from build123d import *

# Parameters (mm, degrees)
CROQUIS1_W              = 150
CROQUIS1_H              = 90
SALIENTE_EXTRUIR1_DEPTH = 5
SALIENTE_EXTRUIR2_DEPTH = 3
CROQUIS2_R              = 2.5
CORTAR_EXTRUIR1_DEPTH   = 10


with BuildPart() as part:
    # Croquis1 → Saliente-Extruir1 (new body)
    with BuildSketch(Plane(origin=(0, 0, 0), x_dir=(1, 0, 0), z_dir=(0, 1, 0))):
        Rectangle(CROQUIS1_W, CROQUIS1_H)
    extrude(amount=SALIENTE_EXTRUIR1_DEPTH)

    # Croquis1<3> → Saliente-Extruir2 (add)
    with BuildSketch(Plane(origin=(0, 0, 0), x_dir=(1, 0, 0), z_dir=(0, 1, 0))):
        Polygon((-75, -45), (-75, 45), (75, 45), (75, -45), (95, -45), (95, 65), (-95, 65), (-95, -45), align=None)
    extrude(amount=SALIENTE_EXTRUIR2_DEPTH)

    # Croquis2 → Cortar-Extruir1 (cut)
    with BuildSketch(Plane.XZ):
        with Locations((85, 30)):
            Circle(CROQUIS2_R)
        with Locations((70, -55)):
            Circle(CROQUIS2_R)
        with Locations((-85, -40)):
            Circle(CROQUIS2_R)
        with Locations((-85, -5)):
            Circle(CROQUIS2_R)
        with Locations((-85, 30)):
            Circle(CROQUIS2_R)
        with Locations((0, -55)):
            Circle(CROQUIS2_R)
        with Locations((-70, -55)):
            Circle(CROQUIS2_R)
        with Locations((85, -5)):
            Circle(CROQUIS2_R)
        with Locations((85, -40)):
            Circle(CROQUIS2_R)
    extrude(amount=-CORTAR_EXTRUIR1_DEPTH, mode=Mode.SUBTRACT)


solid = part.part
Read the model definition and answer for the solid it produces. Units are mm, in the model's axes. Give positions to 0.01 mm unless a question says otherwise; leave off trailing zeros. Write each loop counter-clockwise with the first axis right and the second up, starting at its lowest first coordinate (ties: lowest second). Pieces come first, ordered by that corner, then holes. Notation, with made-up numbers: (57.5, 89) -> (101.5, 89) arc R4 ccw to (101.5, 94) -> close; hole circle Ø3 at (-37, 3). An arc over 180 degrees is marked (long way). Answer as a JSON object with one key per item and string values. Group by question number.
1) Consider L1, parallel to Z at x = -85, y = 1.2; L2, parallel to Z at x = -70, y = 2; L3, parallel to Y at x = -51.5, z = -57.5. Determine where each line is inside the solid, lowest interval first. Write a range as from..to.
2) Each of these flat-tipped pins is pushed along its axis until it touches: P1, Ø1.6, axis at y = 4.5, z = -18, coming from the +X side; P2, Ø4.5, axis at x = 85, z = -5, coming from the -Y side; P3, Ø0.6, axis at y = 3.5, z = 4, coming from the -X side; P4, Ø6, axis at x = -85, z = -5, coming from the +Y side. Where does it stop, or does it pass through?
3) Find section D-D (x = -29). Write down the section's boundary in (y, z).
4) Find section B-B (x = 85). Write down the section's boundary in (y, z), and give its area (3 significant figures).
5) The mould has two halves that part along Z. Classify faces 1 (the cylindrical face through (83, 1.5, -41.5)), 2 (the flat face through (-1, 3, -47)), 3 (the cylindrical face through (-87.5, 1.5, -4.9)), 4 (the flat face through (-1, 2, 45)): +Z half, -Z half, draft (parallel to the pull), parting line (faces both ways), or undercut.
6) Find section A-A (z = -55). Write down the section's boundary in (x, y), and give its area (3 significant figures).
7) Find section C-C (z = 30). Write down the section's boundary in (x, y), and give its area (3 significant figures).
Values follow:
{
 "1": {"L1": "z = -65..-42.5, -37.5..-7.5, -2.5..27.5, 32.5..45", "L2": "z = -65..-57.5, -52.5..45", "L3": "y = 0..3"},
 "2": {"P1": "stops at x = 75", "P2": "passes through", "P3": "stops at x = -75", "P4": "stops at y = 3"},
 "3": {"outline": "(0, -65) -> (3, -65) -> (3, -45) -> (5, -45) -> (5, 45) -> (0, 45) -> close"},
 "4": {"outline": "(0, -65) -> (3, -65) -> (3, -42.5) -> (0, -42.5) -> close; (0, -37.5) -> (3, -37.5) -> (3, -7.5) -> (0, -7.5) -> close; (0, -2.5) -> (3, -2.5) -> (3, 27.5) -> (0, 27.5) -> close; (0, 32.5) -> (3, 32.5) -> (3, 45) -> (0, 45) -> close", "area": "285 mm2"},
 "5": {"face 1": "undercut", "face 2": "draft", "face 3": "undercut", "face 4": "+Z half"},
 "6": {"outline": "(-95, 0) -> (-72.5, 0) -> (-72.5, 3) -> (-95, 3) -> close; (-67.5, 0) -> (-2.5, 0) -> (-2.5, 3) -> (-67.5, 3) -> close; (2.5, 0) -> (67.5, 0) -> (67.5, 3) -> (2.5, 3) -> close; (72.5, 0) -> (95, 0) -> (95, 3) -> (72.5, 3) -> close", "area": "525 mm2"},
 "7": {"outline": "(-95, 0) -> (-87.5, 0) -> (-87.5, 3) -> (-95, 3) -> close; (-82.5, 0) -> (82.5, 0) -> (82.5, 3) -> (75, 3) -> (75, 5) -> (-75, 5) -> (-75, 3) -> (-82.5, 3) -> close; (87.5, 0) -> (95, 0) -> (95, 3) -> (87.5, 3) -> close", "area": "840 mm2"}
}
